```python
from build123d import *

# Parameters (mm, degrees)
SKETCH_W        = 54
SKETCH_H        = 42
SKETCH_W_2      = 44
SKETCH_H_2      = 32
PAD_DEPTH       = 40
SKETCH001_W     = 20
SKETCH001_H     = 5
POCKET_DEPTH    = 40
SKETCH002_R     = 2.5
POCKET001_DEPTH = 42.001
CHAMFER_SIZE    = 1.5
FILLET_R        = 2.5
SKETCH003_R     = 2.5
POCKET002_DEPTH = 42.001
CHAMFER001_SIZE = 1.5
FILLET001_R     = 1.5


with BuildPart() as part:
    # Sketch → Pad (new body)
    with BuildSketch(Plane.XY):
        Rectangle(SKETCH_W, SKETCH_H)
        Rectangle(SKETCH_W_2, SKETCH_H_2, mode=Mode.SUBTRACT)
    extrude(amount=PAD_DEPTH)

    # Sketch001 (on Face10 of Pad) → Pocket (cut)
    with BuildSketch(Plane.XY.offset(40)):
        with Locations((0, 18.5)):
            Rectangle(SKETCH001_W, SKETCH001_H)
    extrude(amount=-POCKET_DEPTH, mode=Mode.SUBTRACT)

    # Sketch002 (on Face14 of Pocket) → Pocket001 (cut, through all)
    with BuildSketch(Plane.XZ.offset(21)):
        with Locations((0, 10)):
            Circle(SKETCH002_R)
    extrude(amount=-POCKET001_DEPTH, mode=Mode.SUBTRACT)

    # Chamfer
    chamfer_edges = [part.edges().sort_by_distance(p)[0] for p in [
        (-2.5, -16, 10),
    ]]
    chamfer(chamfer_edges, length=CHAMFER_SIZE)

    # Fillet
    fillet_edges = [part.edges().sort_by_distance(p)[0] for p in [
        (27, 21, 20),
        (27, 0, 40),
        (-27, 0, 40),
        (-27, 21, 20),
        (-27, 0, 0),
        (27, 0, 0),
        (18.5, 21, 40),
        (-18.5, 21, 40),
        (-18.5, 21, 0),
        (18.5, 21, 0),
    ]]
    fillet(fillet_edges, radius=FILLET_R)

    # Sketch003 (on Face7 of Fillet) → Pocket002 (cut, through all)
    with BuildSketch(Plane.XZ.offset(21)):
        with Locations((0, 30)):
            Circle(SKETCH003_R)
    extrude(amount=-POCKET002_DEPTH, mode=Mode.SUBTRACT)

    # Chamfer001
    chamfer001_edges = [part.edges().sort_by_distance(p)[0] for p in [
        (-2.5, -16, 30),
    ]]
    chamfer(chamfer001_edges, length=CHAMFER001_SIZE)

    # Fillet001
    fillet001_edges = [part.edges().sort_by_distance(p)[0] for p in [
        (-22, 0, 0),
        (0, -16, 0),
        (22, 0, 0),
        (16, 16, 0),
        (-16, 16, 0),
    ]]
    fillet(fillet001_edges, radius=FILLET001_R)


solid = part.part
```
Design review of the part built by this model. Coordinates are the model's own, in mm. A direction names the side the tool comes from. Round coordinates to 2 decimals unless told otherwise and drop trailing zeros. Write each loop counter-clockwise with the first axis right and the second up, starting at its lowest first coordinate (ties: lowest second). Pieces come first, ordered by that corner, then holes.
Item 1: The part is to be moulded in two halves that separate along Y. For faces 1 (the flat face through (-6, -19, 0)), 2 (the flat face through (-16, 16, 20)), 3 (the flat face through (0, -21, 20)), say which applies: +Y half, -Y half, draft (parallel to the pull), parting line (faces both ways), or undercut.
Item 2: Clearance check with a flat-ended pin moving along its axis: pin 1 Ø4.5 at (x, z) = (0, 10) entering from +Y. State where the tip first meets the part, or that it passes through.
Item 3: For faces 4 (the cylindrical face through (0.33, -16.43, 0.45)), 5 (the flat face through (16, 16, 20)), 6 (the flat face through (-10, 18, 20)), list the 3-axis set-ups (+Z, -Z, +X, -X, +Y, -Y) from which the entire face can be reached by the end or side of a thin tool; tool diameter is ignored.
Item 4: We need section C-C on y = -9. Write out the cut boundary in (x, z), and give its area (3 significant figures).
Item 5: We need section B-B on z = 30. Write out the cut boundary in (x, y).
Item 6: For probe 1 along Z at (x, y) = (0, -18.75); probe 2 along X at (y, z) = (17.5, 27); probe 3 along Y at (x, z) = (-19.5, 2.5), list the stretches that pass through material, from the lowest coordinate up.
Item 7: We need section A-A on x = 0. Write out the cut boundary in (y, z), and give its area (3 significant figures).
Item 8: We need section D-D on x = -11.5. Write out the cut boundary in (y, z).
Returned:
1. face 1: draft
1. face 2: undercut
1. face 3: -Y half
2. pin 1: passes through
3. face 4: -Z
3. face 5: +Z, -Z
3. face 6: +Z, -Z, +Y
4. outline: (-27, 2.5) arc R2.5 ccw to (-24.5, 0) - (-23.5, 0) arc R1.5 ccw to (-22, 1.5) - (-22, 40) - (-24.5, 40) arc R2.5 ccw to (-27, 37.5) - close; (22, 1.5) arc R1.5 ccw to (23.5, 0) - (24.5, 0) arc R2.5 ccw to (27, 2.5) - (27, 37.5) arc R2.5 ccw to (24.5, 40) - (22, 40) - close
4. area: 394 mm2
5. outline: (-27, -21) - (-2.5, -21) - (-2.5, -17.5) - (-4, -16) - (-22, -16) - (-22, 16) - (-10, 16) - (-10, 21) - (-24.5, 21) arc R2.5 ccw to (-27, 18.5) - close; (2.5, -21) - (27, -21) - (27, 18.5) arc R2.5 ccw to (24.5, 21) - (10, 21) - (10, 16) - (22, 16) - (22, -16) - (4, -16) - (2.5, -17.5) - close
6. probe 1: z = 0 to 7.5, 12.5 to 27.5, 32.5 to 40
6. probe 2: x = -27 to -10, 10 to 27
6. probe 3: y = -21 to -16, 16 to 21
7. outline: (-21, 0) - (-17.5, 0) arc R1.5 ccw to (-16, 1.5) - (-16, 6) - (-17.5, 7.5) - (-21, 7.5) - close; (-21, 12.5) - (-17.5, 12.5) - (-16, 14) - (-16, 26) - (-17.5, 27.5) - (-21, 27.5) - close; (-21, 32.5) - (-17.5, 32.5) - (-16, 34) - (-16, 40) - (-21, 40) - close
7. area: 145 mm2
8. outline: (-21, 0) - (-17.5, 0) arc R1.5 ccw to (-16, 1.5) - (-16, 40) - (-21, 40) - close; (16, 1.5) arc R1.5 ccw to (17.5, 0) - (18.5, 0) arc R2.5 ccw to (21, 2.5) - (21, 37.5) arc R2.5 ccw to (18.5, 40) - (16, 40) - close
